The listing builds one solid part. Answer for the finished solid, in the listing's coordinates (mm). Face numbers are marked on the shaded views. Coordinates: 2 decimals unless noted, no trailing zeros. Write each loop counter-clockwise with the first axis right and the second up, starting at its lowest first coordinate (ties: lowest second). Pieces come first, ordered by that corner, then holes.
from build123d import *

# Parameters (mm, degrees)
SKETCH037_R         = 6
SKETCH037_R_2       = 2.1
PAD018_DEPTH        = 2
HOLE009_D           = 4.2
HOLE009_DEPTH       = 25
HOLE009_CSINK_D     = 8.2
HOLE009_CSINK_ANGLE = 90


with BuildPart() as part:
    # Sketch037 → Pad018 (new body)
    with BuildSketch(Plane.XY):
        Circle(SKETCH037_R)
        Circle(SKETCH037_R_2, mode=Mode.SUBTRACT)
    extrude(amount=PAD018_DEPTH)

    # Sketch039 (on DatumPlane) → Revolution (revolve)
    with BuildSketch(Plane(origin=(0, 0, 2), x_dir=(1, 0, 0), z_dir=(0, -1, 0))):
        Polygon((2.1, 1.9), (2.1, 0), (4, 0), align=None)
    revolve(axis=Axis((0, 0, 2), (0, 0, 1)))

    # Hole009
    with Locations(Plane(origin=(0, 0, 0), x_dir=(1, 0, 0), z_dir=(0, 0, -1))):
        with Locations((0, 0)):
            CounterSinkHole(HOLE009_D / 2, HOLE009_CSINK_D / 2, depth=HOLE009_DEPTH, counter_sink_angle=HOLE009_CSINK_ANGLE)


solid = part.part
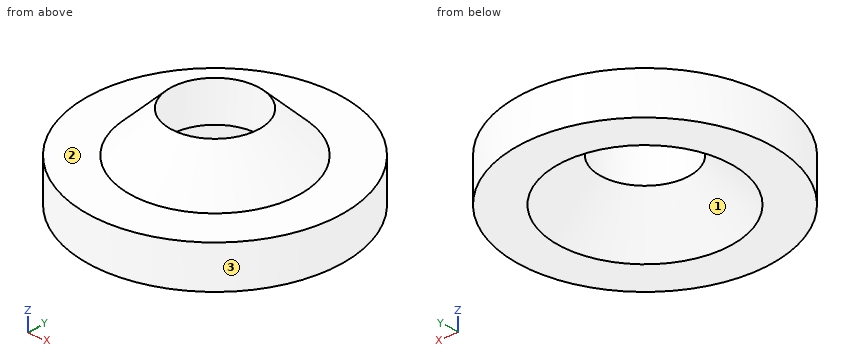
1. Section D-D on y = 5 is taken. Give the vertices of the cut face in (x, z).
Results found:
outline: (-3.32, 0) - (3.32, 0) - (3.32, 2) - (-3.32, 2) - close
2. Find the intervals of material crossed by L1, parallel to Z at x = -4.5, y = 1.25; L2, parallel to Y at x = 0, z = 3; L3, parallel to Y at x = 0, z = 2.55, in increasing order.
Results found:
L1: z = 0 to 2
L2: y = -3 to -2.1, 2.1 to 3
L3: y = -3.45 to -2.1, 2.1 to 3.45
3. For a pull along Y with two mould halves and no side action, classify the marked faces 1, 2 and 3 as pulls with the +Y half, pulls with the -Y half, needs draft (parallel to the pull), parting line crosses it, or undercut.
Results found:
face 1: undercut
face 2: needs draft
face 3: parting line crosses it
4. Section A-A on x = 0 is taken. Give the vertices of the cut face in (y, z), then the cut area to 3 significant figures.
Results found:
outline: (-6, 0) - (-4.1, 0) - (-2.1, 2) - (-2.1, 3.9) - (-4, 2) - (-6, 2) - close; (2.1, 2) - (4.1, 0) - (6, 0) - (6, 2) - (4, 2) - (2.1, 3.9) - close
area: 15.2 mm2
5. Flat-ended cylindrical pins translate along their axes: P1, Ø3, axis at x = -1, y = 4.5, coming from the -Z side; P2, Ø1.5, axis at y = -2, z = 2, coming from the -X side. Find the tip coordinate at first contact, or state that the pin passes through.
Results found:
P1: stops at z = 0
P2: stops at x = -5.87
6. Section C-C on z = 3.25 is taken. Give the vertices of the cut face in (x, y).
Results found:
outline: circle Ø5.5 at (0, 0); hole circle Ø4.2 at (0, 0)
